from build123d import *

# Parameters (mm, degrees)
BOSS_EXTRUDE2_DEPTH = 7
BOSS_EXTRUDE3_DEPTH = 15


with BuildPart() as part:
    # Sketch1 → Boss-Extrude2 (new body)
    with BuildSketch(Plane.XY):
        with BuildLine():
            Line((-41.446212302, -25.123400981), (21.822672825, -14.817519442))
            Line((21.822672825, -14.817519442), (26.489801196, 7.266810726))
            Line((26.489801196, 7.266810726), (34.744303123, 7.266810726))
            Line((34.744303123, 7.266810726), (34.744303123, 11.354641566))
            Line((34.744303123, 11.354641566), (23.2245968, 11.838054321))
            Line((23.2245968, 11.838054321), (22.594616957, 29.052034329))
            Line((22.594616957, 29.052034329), (9.094616957, 29.052034329))
            Line((9.094616957, 29.052034329), (9.094616957, 2.846901584))
            ThreePointArc((9.094616957, 2.846901584), (4.094616957, -2.153098416), (-0.905383043, 2.846901584))
            Line((-0.905383043, 2.846901584), (-0.905383043, 20.539136331))
            Line((-0.905383043, 20.539136331), (-10.036820206, 32.783811613))
            Line((-10.036820206, 32.783811613), (-20.38656022, 37.570023616))
            Line((-20.38656022, 37.570023616), (-22.390510994, 33.236665732))
            Line((-22.390510994, 33.236665732), (-41.446212302, 41.354859092))
            Line((-41.446212302, 41.354859092), (-41.446212302, -25.123400981))
        make_face()
        with BuildLine():
            ThreePointArc((7.629856976, -12.798163857), (7.149099204, -12.884055354), (6.665935601, -12.955177206))
            Line((6.665935601, -12.955177206), (7.629856976, -12.798163857))
        make_face(mode=Mode.SUBTRACT)
    extrude(amount=BOSS_EXTRUDE2_DEPTH)

    # Sketch1_7 → Boss-Extrude3 (add)
    with BuildSketch(Plane.XY):
        with BuildLine():
            Line((-38.38035072, 22.006840878), (-40.987397009, 0.6503843))
            Line((-40.987397009, 0.6503843), (-28.371326411, 4.352577852))
            ThreePointArc((-28.371326411, 4.352577852), (-30.174945318, 4.304423786), (-31.92964529, 4.724409482))
            ThreePointArc((-31.92964529, 4.724409482), (-36.334853416, 11.90193291), (-30.540963199, 18.013686941))
            ThreePointArc((-30.540963199, 18.013686941), (-28.737344292, 18.061841008), (-26.982644321, 17.641855311))
            Line((-26.982644321, 17.641855311), (-38.38035072, 22.006840878))
        make_face()
        with BuildLine():
            Line((-31.92964529, 4.724409482), (-29.456144805, 11.183132397))
            Line((-29.456144805, 11.183132397), (-30.540963199, 18.013686941))
            ThreePointArc((-30.540963199, 18.013686941), (-36.334853416, 11.90193291), (-31.92964529, 4.724409482))
        make_face()
        Polygon((-41.446212302, 0.515744675), (-40.987397009, 0.6503843), (-38.38035072, 22.006840878), (-41.446212302, 23.180975488), align=None)
        with BuildLine():
            Line((-29.456144805, 11.183132397), (-28.371326411, 4.352577852))
            ThreePointArc((-28.371326411, 4.352577852), (-24.196102656, 6.692557499), (-22.539982117, 11.183132397))
            ThreePointArc((-22.539982117, 11.183132397), (-23.757880241, 15.102709834), (-26.982644321, 17.641855311))
            Line((-26.982644321, 17.641855311), (-29.456144805, 11.183132397))
        make_face()
        with BuildLine():
            ThreePointArc((-31.92964529, 4.724409482), (-30.174945318, 4.304423786), (-28.371326411, 4.352577852))
            Line((-28.371326411, 4.352577852), (-29.456144805, 11.183132397))
            Line((-29.456144805, 11.183132397), (-31.92964529, 4.724409482))
        make_face()
        with BuildLine():
            Line((-29.456144805, 11.183132397), (-26.982644321, 17.641855311))
            ThreePointArc((-26.982644321, 17.641855311), (-28.737344292, 18.061841008), (-30.540963199, 18.013686941))
            Line((-30.540963199, 18.013686941), (-29.456144805, 11.183132397))
        make_face()
        with BuildLine():
            Line((-12.043630753, 28.828642478), (-3.015328717, 16.855415173))
            ThreePointArc((-3.015328717, 16.855415173), (-1.977696529, 17.370604665), (-0.905383043, 17.809061684))
            Line((-0.905383043, 17.809061684), (-0.905383043, 20.539136331))
            Line((-0.905383043, 20.539136331), (-7.253856265, 29.052034329))
            Line((-7.253856265, 29.052034329), (-10.036820206, 32.783811613))
            Line((-10.036820206, 32.783811613), (-20.38656022, 37.570023616))
            Line((-20.38656022, 37.570023616), (-22.390510994, 33.236665732))
            Line((-22.390510994, 33.236665732), (-12.043630753, 28.828642478))
        make_face()
        with BuildLine():
            Line((-41.446212302, -20.792174742), (-41.446212302, -25.123400981))
            Line((-41.446212302, -25.123400981), (21.822672825, -14.817519442))
            Line((21.822672825, -14.817519442), (26.489801196, 7.266810726))
            Line((26.489801196, 7.266810726), (34.744303123, 7.266810726))
            Line((34.744303123, 7.266810726), (34.744303123, 11.354641566))
            Line((34.744303123, 11.354641566), (23.2245968, 11.838054321))
            Line((23.2245968, 11.838054321), (22.257186267, 10.122973627))
            Line((22.257186267, 10.122973627), (21.454558852, 7.246323498))
            Line((21.454558852, 7.246323498), (20.850125794, 5.080010211))
            Line((20.850125794, 5.080010211), (20.523303512, 3.077207951))
            ThreePointArc((20.523303512, 3.077207951), (20.524551535, 2.962057773), (20.524967549, 2.846901584))
            ThreePointArc((20.524967549, 2.846901584), (16.885705144, -7.29030648), (7.629856976, -12.798163857))
            ThreePointArc((7.629856976, -12.798163857), (7.149099204, -12.884055354), (6.665935601, -12.955177206))
            Line((6.665935601, -12.955177206), (-1.475395331, -14.281320254))
            Line((-1.475395331, -14.281320254), (-41.446212302, -20.792174742))
        make_face()
    extrude(amount=BOSS_EXTRUDE3_DEPTH)


solid = part.part
Input: part model. Units: mm. Frame: model coordinates. A direction names the side the tool comes from. Coordinates: 2 decimals unless noted, no trailing zeros. Order: outer loops, then holes, each group sorted by start corner. A loop starts at its lowest first (then second) coordinate and runs counter-clockwise, first axis right, second up.
1. Cut plane B-B, the plane y = 36. Return loops of the section in (x, z).
Checked values:
outline: (-41.45, 0) - (-28.88, 0) - (-28.88, 7) - (-41.45, 7) - close; (-21.11, 0) - (-16.99, 0) - (-16.99, 15) - (-21.11, 15) - close
2. Contact query for flat-ended pins moving along their axis: P1, Ø12, axis at x = 17, y = 24.5, coming from the +Z side; P2, Ø18.5, axis at x = -14, y = 12.5, coming from the +Z side; P3, Ø1.5, axis at x = 4.5, z = 5.5, coming from the -Y side; P4, Ø6, axis at x = 13, z = 3.5, coming from the -Y side. Output: stop coordinate, or through.
Checked values:
P1: stops at z = 7
P2: stops at z = 15
P3: stops at y = -17.76
P4: stops at y = -16.74
3. Draft query along Y for faces 4 (the flat face through (-12, 9, 0)), 5 (the flat face through (20.69, 4.09, 10.94)), 6 (the flat face through (-10, -20, 7)), 7 (the flat face through (-7.593, 22.926, 10.944)). Return one class per face: +Y half, -Y half, draft (parallel to the pull), parting line (faces both ways), or undercut.
Checked values:
face 4: draft
face 5: +Y half
face 6: -Y half
face 7: undercut
4. Cut plane C-C, the plane x = 14. Return loops of the section in (y, z).
Checked values:
outline: (-16.09, 0) - (29.05, 0) - (29.05, 7) - (-10.01, 7) - (-10.01, 15) - (-16.09, 15) - close
5. Cut plane D-D, the plane x = -25.5. Return loops of the section in (y, z), plus the area to 3 significant figures.
Checked values:
outline: (-22.53, 0) - (34.56, 0) - (34.56, 7) - (16.86, 7) - (16.86, 15) - (5.51, 15) - (5.51, 7) - (-18.19, 7) - (-18.19, 15) - (-22.53, 15) - close
area: 525 mm2
6. Ray query, line 1 along X through (y, z) = (13.5, 5); line 2 along X through (y, z) = (10, 4); line 3 along Z through (x, y) = (-33, -19). Return the intervals inside material, ascending.
Checked values:
line 1: x = -41.45 to -0.91, 9.09 to 23.16
line 2: x = -41.45 to -0.91, 9.09 to 34.74
line 3: z = 0 to 7
7. Cut plane A-A, the plane z = 8.75. Return loops of the section in (x, y).
Checked values:
outline: (-41.45, -25.12) - (21.82, -14.82) - (26.49, 7.27) - (34.74, 7.27) - (34.74, 11.35) - (23.22, 11.84) - (22.26, 10.12) - (20.85, 5.08) - (20.52, 3.08) arc R15.94 cw to (20.52, 2.85) arc R15.94 cw to (6.67, -12.96) - (-41.45, -20.79) - close; (-41.45, 0.52) - (-28.37, 4.35) arc R6.92 ccw to (-26.98, 17.64) - (-41.45, 23.18) - close; (-22.39, 33.24) - (-12.04, 28.83) - (-3.02, 16.86) arc R15.94 cw to (-0.91, 17.81) - (-0.91, 20.54) - (-10.04, 32.78) - (-20.39, 37.57) - close
8. Access query for faces 1 (the flat face through (-17.289, 31.064, 10.944)), 2 (the flat face through (-31.785, 37.239, 3.451)), 3 (the flat face through (-10, 4, 7)). Directions: +Z, -Z, +X, -X, +Y, -Y. A direction counts if a zero-diameter tool reaches every point of the face in a straight line with its end or side. Return the directions, or none.
Checked values:
face 1: +Z, -X
face 2: +Z, -Z, +Y
face 3: +Z
